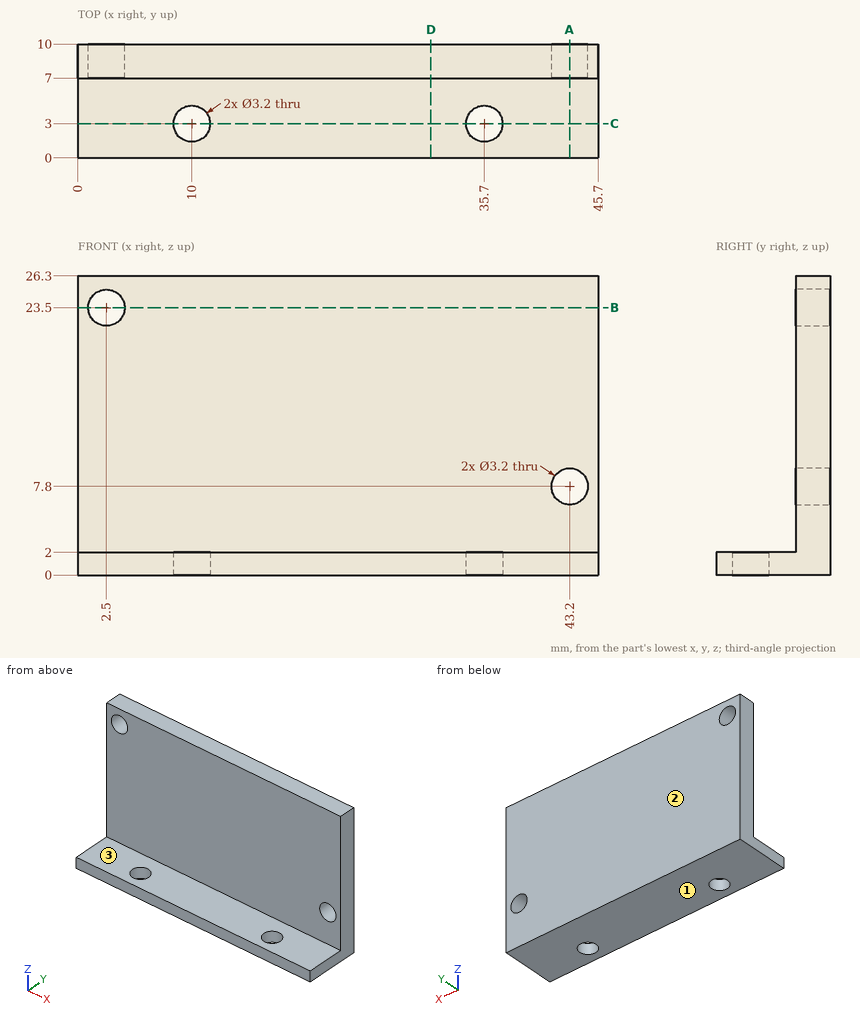
For this review, use the dimensioned drawing (mm, ordinates from the lowest corner) and the shaded views. Coordinates: 2 decimals unless noted, no trailing zeros. Loops run counter-clockwise (first coordinate to the right, second up) from the corner with the lowest first, then second, coordinate; pieces in that order, holes last.
1. Add section A-A, the plane x = 43.2. Give the boundary of the cut face in (y, z), then the cut area to 3 significant figures.
2. Insertion check: P1, Ø10, axis at x = 36.5, z = 21, coming from the -Y side; P2, Ø3, axis at x = 35.7, y = 3, coming from the +Z side (3 decimals); P3, Ø5, axis at x = 23, y = 4, coming from the +Z side. Each pin has a flat end and moves straight along its axis. Give the tip position at first contact, or say it passes through.
3. Add section D-D, the plane x = 31. Give the boundary of the cut face in (y, z).
4. Add section C-C, the plane y = 3. Give the boundary of the cut face in (x, z), then the cut area to 3 significant figures.
5. Mouldability with a two-part tool opening along Z and no side actions: class the marked faces 1, 2 and 3 as +Z half, -Z half, draft (parallel to the pull), parting line (faces both ways), or undercut.
6. Add section B-B, the plane z = 23.5. Give the boundary of the cut face in (x, y).
7. For line 1 (X direction, y = 8.35, z = 7.8); line 2 (Y direction, x = 35.7, z = 1.35); line 3 (Z direction, x = 31, y = 5.75), list the stretches that pass through material, from the lowest coordinate up.
Result:
1. outline: (0, 0) - (10, 0) - (10, 6.2) - (7, 6.2) - (7, 2) - (0, 2) - close; (7, 9.4) - (10, 9.4) - (10, 26.3) - (7, 26.3) - close
1. area: 83.3 mm2
2. P1: stops at y = 7
2. P2: passes through
2. P3: stops at z = 2
3. outline: (0, 0) - (10, 0) - (10, 26.3) - (7, 26.3) - (7, 2) - (0, 2) - close
4. outline: (0, 0) - (8.4, 0) - (8.4, 2) - (0, 2) - close; (11.6, 0) - (34.1, 0) - (34.1, 2) - (11.6, 2) - close; (37.3, 0) - (45.7, 0) - (45.7, 2) - (37.3, 2) - close
4. area: 78.6 mm2
5. face 1: -Z half
5. face 2: draft
5. face 3: +Z half
6. outline: (0, 7) - (0.9, 7) - (0.9, 10) - (0, 10) - close; (4.1, 7) - (45.7, 7) - (45.7, 10) - (4.1, 10) - close
7. line 1: x = 0 to 41.6, 44.8 to 45.7
7. line 2: y = 0 to 1.4, 4.6 to 10
7. line 3: z = 0 to 2
